```python
from build123d import *

# Parameters (mm, degrees)
SKETCH1_R           = 12.5
BOSS_EXTRUDE1_DEPTH = 20
SKETCH2_R           = 7.5
BOSS_EXTRUDE2_DEPTH = 20
SKETCH3_R           = 17.5
BOSS_EXTRUDE3_DEPTH = 10
SKETCH4_R           = 4
BOSS_EXTRUDE4_DEPTH = 215
SKETCH5_W           = 12
SKETCH5_H           = 4
CUT_EXTRUDE1_DEPTH  = 6
SKETCH6_R           = 1
BOSS_EXTRUDE5_DEPTH = 4


with BuildPart() as part:
    # Sketch1 → Boss-Extrude1 (new body)
    with BuildSketch(Plane(origin=(0, 0, 0), x_dir=(0, 0, -1), z_dir=(1, 0, 0))):
        Circle(SKETCH1_R)
    extrude(amount=BOSS_EXTRUDE1_DEPTH)

    # Sketch2 → Boss-Extrude2 (add)
    with BuildSketch(Plane(origin=(20, 0, 0), x_dir=(0, 0, -1), z_dir=(1, 0, 0))):
        Circle(SKETCH2_R)
    extrude(amount=BOSS_EXTRUDE2_DEPTH)

    # Sketch3 → Boss-Extrude3 (add)
    with BuildSketch(Plane(origin=(40, 0, 0), x_dir=(0, 0, -1), z_dir=(1, 0, 0))):
        Circle(SKETCH3_R)
    extrude(amount=BOSS_EXTRUDE3_DEPTH)

    # Sketch4 → Boss-Extrude4 (add)
    with BuildSketch(Plane(origin=(50, 0, 0), x_dir=(0, 0, -1), z_dir=(1, 0, 0))):
        Circle(SKETCH4_R)
    extrude(amount=BOSS_EXTRUDE4_DEPTH)

    # Sketch5 → Cut-Extrude1 (cut)
    with BuildSketch(Plane(origin=(265, 0, 0), x_dir=(0, 0, -1), z_dir=(1, 0, 0))):
        Rectangle(SKETCH5_W, SKETCH5_H)
    extrude(amount=-CUT_EXTRUDE1_DEPTH, mode=Mode.SUBTRACT)

    # Sketch6 → Boss-Extrude5 (add)
    with BuildSketch(Plane(origin=(0, -2, 0), x_dir=(1, 0, 0), z_dir=(0, 1, 0))):
        with Locations(Location((262, 0, 0), (0, 0, 90))):
            Circle(SKETCH6_R)
    extrude(amount=BOSS_EXTRUDE5_DEPTH)


solid = part.part
```
The model under review builds one solid part; all positions refer to its coordinate system, in mm. A direction names the side the tool comes from. Give positions to 0.01 mm unless a question says otherwise; leave off trailing zeros. Write each loop counter-clockwise with the first axis right and the second up, starting at its lowest first coordinate (ties: lowest second). Pieces come first, ordered by that corner, then holes. Notation, with made-up numbers: (-3.75, 20) - (10.25, 20) arc R19 cw to (10.25, 34) - close; hole circle Ø10 at (82.25, 87.25). An arc over 180 degrees is marked (long way). Answer in a Markdown table with one row per item. Add a question column.
1. Draft analysis for pull direction X (two halves, no side actions). For faces 1 (the flat face through (40, -8, 0)), 2 (the flat face through (0, 0, 0)), 3 (the cylindrical face through (9.86, 3.755, -11.923)), 4 (the cylindrical face through (29.86, 0.33, 7.493)), state which applies: +X half, -X half, draft (parallel to the pull), parting line (faces both ways), or undercut.
2. Wall thickness on line 1 along X through (y, z) = (-10.5, -2); line 2 along Y through (x, z) = (131.5, 2); line 3 along Z through (x, y) = (198, 0.5): over which ranges is each line inside the solid? List them lowest first. Write a range as [from, to].
3. Insertion check: P1, Ø3, axis at x = 260.5, z = -1.5, coming from the +Y side; P2, Ø12, axis at x = 87.5, z = 8, coming from the -Y side; P3, Ø8, axis at x = 226, y = -0.5, coming from the +Z side. Each pin has a flat end and moves straight along its axis. Give the tip position at first contact, or say it passes through.
4. Tool access review of faces 5 (the cylindrical face through (44.93, -10.648, 13.887)), 6 (the flat face through (263, 2, 1)), 7 (the cylindrical face through (155.995, -3.905, 0.867)): name each direction out of +Z, -Z, +X, -X, +Y, -Y from which nothing blocks a thin tool from reaching the whole face with its end or side.
5. We need section A-A on x = 203. Write out the cut boundary in (y, z), then the cut area to 3 significant figures.
6. We need section B-B on y = 15. Write out the cut boundary in (x, z).
Ans:
| question | item | result |
|---|---|---|
| 1 | face 1 | undercut |
| 1 | face 2 | -X half |
| 1 | face 3 | draft |
| 1 | face 4 | undercut |
| 2 | line 1 | x = [0, 20], [40, 50] |
| 2 | line 2 | y = [-3.46, 3.46] |
| 2 | line 3 | z = [-3.97, 3.97] |
| 3 | P1 | stops at y = 4 |
| 3 | P2 | stops at y = -3.46 |
| 3 | P3 | stops at z = 4 |
| 4 | face 5 | +X, -X |
| 4 | face 6 | none |
| 4 | face 7 | +X |
| 5 | outline | circle Ø8 at (0, 0) |
| 5 | area | 50.3 mm^2 |
| 6 | outline | (40, -9.01) - (50, -9.01) - (50, 9.01) - (40, 9.01) - close |
